```python
from build123d import *

# Parameters (mm, degrees)
SKETCH2_R                       = 80
SKETCH2_R_2                     = 31
BOSS_EXTRUDE1_DEPTH             = 5
F_4_0MM_DOWEL_HOLE1_D           = 4
F_4_0MM_DOWEL_HOLE1_CSINK_D     = 4.05
F_4_0MM_DOWEL_HOLE1_CSINK_ANGLE = 90
F_3_0MM_DOWEL_HOLE1_D           = 3
F_3_0MM_DOWEL_HOLE1_CSINK_D     = 3.05
F_3_0MM_DOWEL_HOLE1_CSINK_ANGLE = 90


with BuildPart() as part:
    # Sketch2 → Boss-Extrude1 (new body)
    with BuildSketch(Plane.XY):
        Circle(SKETCH2_R)
        Circle(SKETCH2_R_2, mode=Mode.SUBTRACT)
    extrude(amount=BOSS_EXTRUDE1_DEPTH)

    # Ø4.0mm Dowel Hole1 (through all)
    with Locations(Plane.XY.offset(5)):
        with Locations((0, 70), (-49.497474683, 49.497474683), (-70, 0), (-49.497474683, -49.497474683), (0, -70), (49.497474683, -49.497474683), (70, 0), (49.497474683, 49.497474683)):
            CounterSinkHole(F_4_0MM_DOWEL_HOLE1_D / 2, F_4_0MM_DOWEL_HOLE1_CSINK_D / 2, counter_sink_angle=F_4_0MM_DOWEL_HOLE1_CSINK_ANGLE)

    # Ø3.0mm Dowel Hole1 (through all)
    with Locations(Plane.XY.offset(5)):
        with Locations((0, 37), (-26.162950904, 26.162950904), (-37, 0), (-26.162950904, -26.162950904), (0, -37), (26.162950904, -26.162950904), (37, 0), (26.162950904, 26.162950904)):
            CounterSinkHole(F_3_0MM_DOWEL_HOLE1_D / 2, F_3_0MM_DOWEL_HOLE1_CSINK_D / 2, counter_sink_angle=F_3_0MM_DOWEL_HOLE1_CSINK_ANGLE)


solid = part.part
```
The listing builds one solid part. Answer for the finished solid, in the listing's coordinates (mm). Round coordinates to 2 decimals unless told otherwise and drop trailing zeros. Loops run counter-clockwise (first coordinate to the right, second up) from the corner with the lowest first, then second, coordinate; pieces in that order, holes last. Notation, with made-up numbers: (42.5, 13.5) - (96.5, 13.5) arc R11 ccw to (96.5, 28.5) - close; hole circle Ø8 at (-0.5, 9). An arc over 180 degrees is marked (long way). Return JSON: item names as keys, results as strings. Group by question number.
1. Each of these flat-tipped pins is pushed along its axis until it touches: P1, Ø1.5, axis at x = -5.5, z = 2, coming from the -Y side; P2, Ø2, axis at y = -62.5, z = 0.5, coming from the +X side; P3, Ø3, axis at y = -2.5, z = 4.5, coming from the -X side. Where does it stop, or does it pass through?
2. The mould has two halves that part along X. Classify faces 1 (the cylindrical face through (-17.34, -78.1, 2.46)), 2 (the cylindrical face through (47.59, 50.1, 2.45)), 3 (the flat face through (-1, -34, 5)): pulls with the +X half, pulls with the -X half, needs draft (parallel to the pull), parting line crosses it, or undercut.
3. Consider probe 1 along Y at (x, z) = (0, 4); probe 2 along Y at (x, z) = (-50.5, 3.6); probe 3 along Y at (x, z) = (-51, 2). Determine where each line is inside the solid, lowest interval first.
4. The part is cut by section C-C on z = 2.4. State how many separate pieces and enclosed holes the cut face has, then the cut area to 3 significant figures.
5. The part is cut by section A-A on y = -13.5. Determine the outline of the cut face in (x, z).
6. The part is cut by section B-B on x = -70. Determine the outline of the cut face in (y, z) (3 decimals).
7. The part is cut by section D-D on y = 11.5. Determine the outline of the cut face in (x, z).
Resolved:
{
 "1": {"P1": "stops at y = -79.86", "P2": "stops at x = 51.16", "P3": "stops at x = -79.99"},
 "2": {"face 1": "parting line crosses it", "face 2": "undercut", "face 3": "needs draft"},
 "3": {"probe 1": "y = -80 to -72, -68 to -38.5, -35.5 to -31, 31 to 35.5, 38.5 to 68, 72 to 80", "probe 2": "y = -62.05 to -51.23, -47.77 to 47.77, 51.23 to 62.05", "probe 3": "y = -61.64 to -50.82, -48.18 to 48.18, 50.82 to 61.64"},
 "4": {"separate pieces": "1", "enclosed holes": "17", "area": "16,900 mm²"},
 "5": {"outline": "(-78.85, 0) - (-27.91, 0) - (-27.91, 5) - (-78.85, 5) - close; (27.91, 0) - (78.85, 0) - (78.85, 5) - (27.91, 5) - close"},
 "6": {"outline": "(-38.73, 0) - (-2, 0) - (-2, 4.975) - (-2.025, 5) - (-38.73, 5) - close; (2, 0) - (38.73, 0) - (38.73, 5) - (2.025, 5) - (2, 4.975) - close"},
 "7": {"outline": "(-79.17, 0) - (-28.79, 0) - (-28.79, 5) - (-79.17, 5) - close; (28.79, 0) - (79.17, 0) - (79.17, 5) - (28.79, 5) - close"}
}
